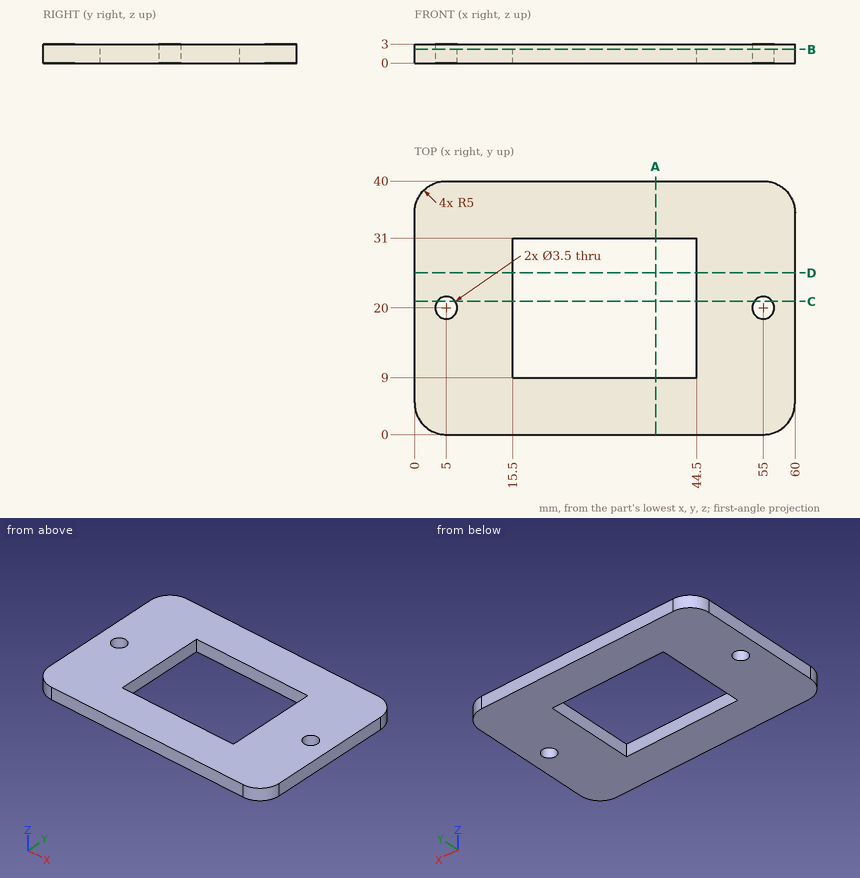
Study the drawing (mm; zero at the part's minimum x, y, z) and answer. Give positions to 0.01 mm unless a question says otherwise; leave off trailing zeros. Write each loop counter-clockwise with the first axis right and the second up, starting at its lowest first coordinate (ties: lowest second). Pieces come first, ordered by that corner, then holes. Notation, with made-up numbers: (-22.5, 76.25) -> (12.5, 76.25) arc R19 cw to (12.5, 100.25) -> close; hole circle Ø4 at (21, 57). An arc over 180 degrees is marked (long way). Write item = value, one per line. Start each with the question number.
1) The part is cut by section B-B, the plane z = 2.15. Determine the outline of the cut face in (x, y), and give its area (3 significant figures).
2) The part is cut by section C-C, the plane y = 21. Determine the outline of the cut face in (x, z), and give its area (3 significant figures).
3) Straight lines are drawn through the part: line 1 along X through (y, z) = (11, 2.2); line 2 along Y through (x, z) = (27, 1.45); line 3 along X through (y, z) = (19, 1.2). For each, find the intervals that lie inside material, in ascending order.
4) Each of these flat-tipped pins is pushed along its axis until it touches: pin 1 (5 mm diameter, centred on x = 7, y = 9, fed in from -Z); pin 2 (3 mm diameter, centred on x = 55, y = 20, fed in from +Z). Where does it stop, or does it pass through?
5) The part is cut by section D-D, the plane y = 25.5. Determine the outline of the cut face in (x, z).
6) The part is cut by section A-A, the plane x = 38. Determine the outline of the cut face in (y, z), and give its area (3 significant figures).
Solutions:
q1.outline = (0, 5) arc R5 ccw to (5, 0) -> (55, 0) arc R5 ccw to (60, 5) -> (60, 35) arc R5 ccw to (55, 40) -> (5, 40) arc R5 ccw to (0, 35) -> close; hole circle Ø3.5 at (5, 20); hole (15.5, 9) -> (44.5, 9) -> (44.5, 31) -> (15.5, 31) -> close; hole circle Ø3.5 at (55, 20)
q1.area = 1,720 mm²
q2.outline = (0, 0) -> (3.56, 0) -> (3.56, 3) -> (0, 3) -> close; (6.44, 0) -> (15.5, 0) -> (15.5, 3) -> (6.44, 3) -> close; (44.5, 0) -> (53.56, 0) -> (53.56, 3) -> (44.5, 3) -> close; (56.44, 0) -> (60, 0) -> (60, 3) -> (56.44, 3) -> close
q2.area = 75.8 mm²
q3.line_1 = 0 to 15.5, 44.5 to 60
q3.line_2 = 0 to 9, 31 to 40
q3.line_3 = 0 to 3.56, 6.44 to 15.5, 44.5 to 53.56, 56.44 to 60
q4.pin_1 = 0
q4.pin_2 = through
q5.outline = (0, 0) -> (15.5, 0) -> (15.5, 3) -> (0, 3) -> close; (44.5, 0) -> (60, 0) -> (60, 3) -> (44.5, 3) -> close
q6.outline = (0, 0) -> (9, 0) -> (9, 3) -> (0, 3) -> close; (31, 0) -> (40, 0) -> (40, 3) -> (31, 3) -> close
q6.area = 54.0 mm²
